from build123d import *

# Parameters (mm, degrees)
RESSALTO_EXTRUS_O4_DEPTH = 5
RESSALTO_EXTRUS_O6_DEPTH = 102
ESBO_O9_W                = 52
ESBO_O9_H                = 5
RESSALTO_EXTRUS_O7_DEPTH = 45
ESBO_O10_R               = 2.25
CORTE_EXTRUS_O1_DEPTH    = 103
FILETE1_R                = 3
FILETE3_R                = 2
FILETE5_R                = 2
ESBO_O11_R               = 1.75
ESBO_O11_W               = 28.2
ESBO_O11_H               = 54.2
CORTE_EXTRUS_O2_DEPTH    = 46
CORTE_EXTRUS_O3_DEPTH    = 46
CHANFRO1_SIZE            = 1


with BuildPart() as part:
    # Esboço7 → Ressalto-extrusão4 (new body)
    with BuildSketch(Plane(origin=(0, 0, 0), x_dir=(1, 0, 0), z_dir=(0, 1, 0))):
        Polygon((21, 45), (21, 5), (-21, 5), (-21, 45), (-41, 45), (-41, 0), (41, 0), (41, 45), align=None)
    extrude(amount=RESSALTO_EXTRUS_O4_DEPTH)

    # Esboço8 → Ressalto-extrusão6 (add)
    with BuildSketch(Plane(origin=(0, 0, 0), x_dir=(1, 0, 0), z_dir=(0, 1, 0))):
        Polygon((-21, 45), (-26, 45), (-26, 0), (26, 0), (26, 45), (21, 45), (21, 5), (-21, 5), align=None)
    extrude(amount=RESSALTO_EXTRUS_O6_DEPTH)

    # Esboço9 → Ressalto-extrusão7 (add)
    with BuildSketch(Plane.XY):
        with Locations((0, 99.5)):
            Rectangle(ESBO_O9_W, ESBO_O9_H)
    extrude(amount=-RESSALTO_EXTRUS_O7_DEPTH)

    # Esboço10 → Corte-extrusão1 (cut, through all)
    with BuildSketch(Plane(origin=(0, 0, 0), x_dir=(1, 0, 0), z_dir=(0, 1, 0))):
        with Locations((-33.5, 33.75)):
            Circle(ESBO_O10_R)
        with Locations((-33.5, 11.25)):
            Circle(ESBO_O10_R)
        with Locations((33.5, 11.25)):
            Circle(ESBO_O10_R)
        with Locations((33.5, 33.75)):
            Circle(ESBO_O10_R)
    extrude(amount=CORTE_EXTRUS_O1_DEPTH, mode=Mode.SUBTRACT)

    # Filete1
    filete1_edges = [part.edges().sort_by_distance(p)[0] for p in [
        (-26, 5, -22.5),
        (26, 5, -22.5),
    ]]
    fillet(filete1_edges, radius=FILETE1_R)

    # Filete3
    filete3_edges = [part.edges().sort_by_distance(p)[0] for p in [
        (41, 2.5, 0),
        (-41, 2.5, 0),
        (-41, 2.5, -45),
        (41, 2.5, -45),
    ]]
    fillet(filete3_edges, radius=FILETE3_R)

    # Filete5
    filete5_edges = [part.edges().sort_by_distance(p)[0] for p in [
        (-26, 102, -22.5),
        (26, 102, -22.5),
    ]]
    fillet(filete5_edges, radius=FILETE5_R)

    # Esboço11 → Corte-extrusão2 (cut, through all)
    with BuildSketch(Plane.XY):
        with Locations((20, 32.1)):
            Circle(ESBO_O11_R)
        with Locations((-20, 32.1)):
            Circle(ESBO_O11_R)
        with Locations((0, 32.1)):
            Rectangle(ESBO_O11_W, ESBO_O11_H)
    extrude(amount=-CORTE_EXTRUS_O2_DEPTH, mode=Mode.SUBTRACT)

    # Esboço12 → Corte-extrusão3 (cut, through all)
    with BuildSketch(Plane.XY):
        with BuildLine():
            Line((-17.5, 100.1), (17.5, 100.1))
            ThreePointArc((17.5, 100.1), (19.5, 98.1), (17.5, 96.1))
            Line((17.5, 96.1), (-17.5, 96.1))
            ThreePointArc((-17.5, 96.1), (-19.5, 98.1), (-17.5, 100.1))
        make_face()
        with BuildLine():
            Line((-17.5, 93.1), (17.5, 93.1))
            ThreePointArc((17.5, 93.1), (19.5, 91.1), (17.5, 89.1))
            Line((17.5, 89.1), (-17.5, 89.1))
            ThreePointArc((-17.5, 89.1), (-19.5, 91.1), (-17.5, 93.1))
        make_face()
        with BuildLine():
            Line((-17.5, 86.1), (17.5, 86.1))
            ThreePointArc((17.5, 86.1), (19.5, 84.1), (17.5, 82.1))
            Line((17.5, 82.1), (-17.5, 82.1))
            ThreePointArc((-17.5, 82.1), (-19.5, 84.1), (-17.5, 86.1))
        make_face()
        with BuildLine():
            Line((-17.5, 79.1), (17.5, 79.1))
            ThreePointArc((17.5, 79.1), (19.5, 77.1), (17.5, 75.1))
            Line((17.5, 75.1), (-17.5, 75.1))
            ThreePointArc((-17.5, 75.1), (-19.5, 77.1), (-17.5, 79.1))
        make_face()
        with BuildLine():
            Line((-17.5, 72.1), (17.5, 72.1))
            ThreePointArc((17.5, 72.1), (19.5, 70.1), (17.5, 68.1))
            Line((17.5, 68.1), (-17.5, 68.1))
            ThreePointArc((-17.5, 68.1), (-19.5, 70.1), (-17.5, 72.1))
        make_face()
        with BuildLine():
            Line((-17.5, 65.1), (17.5, 65.1))
            ThreePointArc((17.5, 65.1), (19.5, 63.1), (17.5, 61.1))
            Line((17.5, 61.1), (-17.5, 61.1))
            ThreePointArc((-17.5, 61.1), (-19.5, 63.1), (-17.5, 65.1))
        make_face()
    extrude(amount=-CORTE_EXTRUS_O3_DEPTH, mode=Mode.SUBTRACT)

    # Chanfro1
    chanfro1_edges = [part.edges().sort_by_distance(p)[0] for p in [
        (31.25, 5, -33.75),
        (31.25, 5, -11.25),
        (-35.75, 5, -11.25),
        (-35.75, 5, -33.75),
    ]]
    chamfer(chanfro1_edges, length=CHANFRO1_SIZE)


solid = part.part
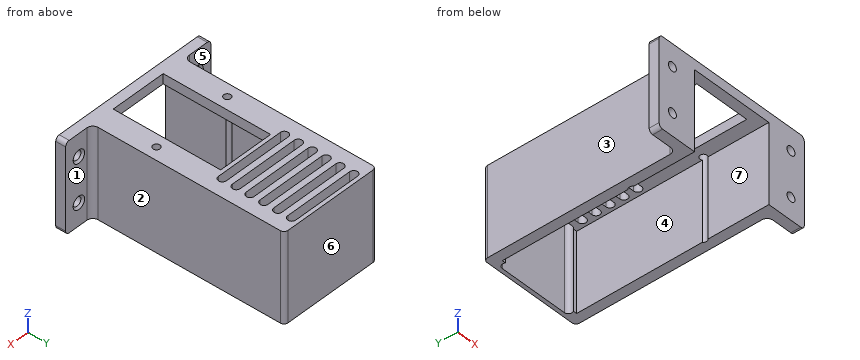
Check sheet for the modelled part. Datum: model origin and axes. Units: mm. Face numbers are marked on the shaded views. A direction names the side the tool comes from. Give positions to 0.01 mm unless a question says otherwise; leave off trailing zeros. Write each loop counter-clockwise with the first axis right and the second up, starting at its lowest first coordinate (ties: lowest second). Pieces come first, ordered by that corner, then holes. Notation, with made-up numbers: (66.25, 65) -> (107.25, 65) arc R23 cw to (107.25, 81) -> close; hole circle Ø8 at (1, -32.75). An arc over 180 degrees is marked (long way). Use one line per item in the form item = value. Start each with the question number.
1. Section check A-A (x = -10). Count the separate pieces of the cut face and the enclosed holes in it, and give its area (3 significant figures).
2. Mould release check, pull along X, two halves, no side actions. Record for the marked faces 1, 2, 3 and 4: pulls with the +X half, pulls with the -X half, needs draft (parallel to the pull), parting line crosses it, or undercut.
3. Section check C-C (z = -6.5). Record the cut outline in (x, y).
4. Access from +Z, -Z, +X, -X, +Y, -Y to the whole of each face (thin tool, end or side, straight path). Record for the marked faces 5, 6 and 7.
5. Go/stop test with flat-tipped pins: P1, Ø1, axis at y = 83, z = -19.5, coming from the -X side; P2, Ø2, axis at y = 18, z = -4.5, coming from the +X side; P3, Ø13, axis at x = -36.5, z = -23, coming from the +Y side; P4, Ø3.5, axis at x = -33.5, z = -33.75, coming from the +Y side. Record where each tip stops, or that it passes through.
6. Thickness scan on line 1 along X through (y, z) = (2.35, -11.25); line 2 along Z through (x, y) = (33.5, 2.8); line 3 along X through (y, z) = (32.1, -30). Record the ranges inside material, lowest first. Write a range as from..to.
7. Section check B-B (y = 77.1). Record the cut outline in (x, z).
Conclusion:
q1.separate_pieces = 8
q1.enclosed_holes = 0
q1.area = 195 mm²
q2.face_1 = needs draft
q2.face_2 = pulls with the +X half
q2.face_3 = pulls with the -X half
q2.face_4 = undercut
q3.outline = (-41, 0) -> (-21, 0) -> (-21, 30.66) arc R1.75 cw to (-21, 33.54) -> (-21, 97) -> (-19.17, 97) arc R2 cw to (-17.5, 100.1) -> (17.5, 100.1) arc R2 cw to (19.17, 97) -> (21, 97) -> (21, 33.54) arc R1.75 cw to (21, 30.66) -> (21, 0) -> (41, 0) -> (41, 5) -> (29, 5) arc R3 cw to (26, 8) -> (26, 100) arc R2 ccw to (24, 102) -> (-24, 102) arc R2 ccw to (-26, 100) -> (-26, 8) arc R3 cw to (-29, 5) -> (-41, 5) -> close
q4.face_5 = +Z, -Z, -X, +Y
q4.face_6 = +Z, -Z, +X, -X, +Y
q4.face_7 = -Z, -Y
q5.P1 = -26
q5.P2 = 26
q5.P3 = 5
q5.P4 = through
q6.line_1 = -41..-35.75, -31.25..-21, 21..31.25, 35.75..41
q6.line_2 = -45..-36, -31.5..-13.5, -9..0
q6.line_3 = -26..-21.75, 21.75..26
q7.outline = (-26, -45) -> (-21, -45) -> (-21, -5) -> (-19.5, -5) -> (-19.5, 0) -> (-26, 0) -> close; (19.5, -5) -> (21, -5) -> (21, -45) -> (26, -45) -> (26, 0) -> (19.5, 0) -> close
